from build123d import *

# Parameters (mm, degrees)
PAD_DEPTH            = 6.5
POCKET_DEPTH         = 6
SKETCH002_R          = 13.5
POCKET001_DEPTH      = 1
SKETCH003_W          = 5.45
SKETCH003_H          = 6.5
PAD001_DEPTH         = 3.5
POCKET002_DEPTH      = 10
SKETCH010_W          = 4
SKETCH010_H          = 6.5
PAD002_DEPTH         = 3.5
POCKET005_DEPTH      = 10
SKETCH015_R          = 2.2
SKETCH015_R_2        = 1.025
PAD003_DEPTH         = 2
POCKET009_DEPTH      = 4
POCKET010_DEPTH      = 4
PAD004_DEPTH         = 4
POCKET013_DEPTH      = 12.201
POCKET013_DEPTH_BACK = 36.201
SKETCH022_R          = 0.6
POCKET014_DEPTH      = 2
SKETCH023_R          = 0.6
POCKET015_DEPTH      = 2
SKETCH024_R          = 13.5
PAD005_DEPTH         = 1
SKETCH025_R          = 20.45
SKETCH025_R_2        = 19.85
POCKET016_DEPTH      = 0.3
SKETCH026_R          = 1
POCKET017_DEPTH      = 5


with BuildPart() as part:
    # Sketch → Pad (new body)
    with BuildSketch(Plane.XY):
        with BuildLine():
            Line((-22.5019915649, 16), (-22.5019915649, -16))
            Line((-22.5019915649, -16), (-16.2858834578, -17.9))
            ThreePointArc((-16.2858834578, -17.9), (-0.4552796053, -24.1957169863), (15.6009615088, -18.5))
            Line((15.6009615088, -18.5), (24.5395016581, -17.45))
            Line((24.5395016581, 17.45), (24.5395016581, -17.45))
            Line((15.6009615088, 18.5), (24.5395016581, 17.45))
            ThreePointArc((15.6009615088, 18.5), (-0.4552796053, 24.1957169863), (-16.2858834578, 17.9))
            Line((-22.5019915649, 16), (-16.2858834578, 17.9))
        make_face()
    extrude(amount=PAD_DEPTH)

    # Sketch001 → Pocket (cut)
    with BuildSketch(Plane.XY):
        with BuildLine():
            Line((-14.8539557021, 16.9), (-21.2122180433, 15.55))
            Line((-21.2122180433, 15.55), (-21.2122180433, -15.55))
            Line((-21.2122180433, -15.55), (-14.8539557021, -16.9))
            ThreePointArc((-14.8539557021, -16.9), (-0.0760301383, -22.4998715423), (14.739402973, -17))
            Line((14.739402973, -17), (23.6191552218, -16.4))
            Line((23.6191552218, 16.4), (23.6191552218, -16.4))
            Line((14.739402973, 17), (23.6191552218, 16.4))
            ThreePointArc((14.739402973, 17), (-0.0760301383, 22.4998715423), (-14.8539557021, 16.9))
        make_face()
    extrude(amount=POCKET_DEPTH, mode=Mode.SUBTRACT)

    # Sketch002 (on Face19 of Pocket) → Pocket001 (cut)
    with BuildSketch(Plane(origin=(0, 0, 6), x_dir=(1, 0, 0), z_dir=(0, 0, -1))):
        Circle(SKETCH002_R)
    extrude(amount=-POCKET001_DEPTH, mode=Mode.SUBTRACT)

    # Sketch003 (on Face7 of Pad) → Pad001 (join)
    with BuildSketch(Plane.YZ.offset(24.5395016581)):
        with Locations((-14.725, 3.25)):
            Rectangle(SKETCH003_W, SKETCH003_H)
        with Locations((14.725, 3.25)):
            Rectangle(SKETCH003_W, SKETCH003_H)
    extrude(amount=PAD001_DEPTH)

    # Sketch006 (on Face22 of Pad001) → Pocket002 (cut)
    with BuildSketch(Plane.XY.offset(6.5)):
        with BuildLine():
            ThreePointArc((24.5395016581, 17.45), (26.1592830786, 16.2095505764), (28.0395016581, 15.4176006311))
            Line((28.0395016581, 17.45), (28.0395016581, 15.4176006311))
            Line((28.0395016581, 17.45), (24.5395016581, 17.45))
        make_face()
        with BuildLine():
            ThreePointArc((28.0395016581, -15.4176006311), (26.1592830786, -16.2095505765), (24.5395016581, -17.4500000001))
            Line((28.0395016581, -17.45), (24.5395016581, -17.4500000001))
            Line((28.0395016581, -15.4176006311), (28.0395016581, -17.45))
        make_face()
    extrude(amount=-POCKET002_DEPTH, mode=Mode.SUBTRACT)

    # Sketch010 (on Face3 of Pad) → Pad002 (join)
    with BuildSketch(Plane(origin=(-22.5019915649, 0, 0), x_dir=(0, -1, 0), z_dir=(-1, 0, 0))):
        with Locations((-14, 3.25)):
            Rectangle(SKETCH010_W, SKETCH010_H)
        with Locations((14, 3.25)):
            Rectangle(SKETCH010_W, SKETCH010_H)
    extrude(amount=PAD002_DEPTH)

    # Sketch011 (on Face28 of Pad002) → Pocket005 (cut)
    with BuildSketch(Plane.XY.offset(6.5)):
        Polygon((-26.0019915649, 16), (-22.5019915649, 16), (-26.0019915649, 14.5), align=None)
        Polygon((-22.5019915649, -16), (-26.0019915649, -14.5), (-26.0019915649, -16), align=None)
    extrude(amount=-POCKET005_DEPTH, mode=Mode.SUBTRACT)

    # Sketch015 (on Face19 of Pocket) → Pad003 (join)
    with BuildSketch(Plane(origin=(0, 0, 6), x_dir=(1, 0, 0), z_dir=(0, 0, -1))):
        with Locations((-18.42, 13.32)):
            Circle(SKETCH015_R)
        with Locations((-18.42, 13.32)):
            Circle(SKETCH015_R_2, mode=Mode.SUBTRACT)
        with Locations((7.27, 18.56)):
            Circle(SKETCH015_R)
        with Locations((7.27, 18.56)):
            Circle(SKETCH015_R_2, mode=Mode.SUBTRACT)
        with Locations((5.37, -19.79)):
            Circle(SKETCH015_R)
        with Locations((5.37, -19.79)):
            Circle(SKETCH015_R_2, mode=Mode.SUBTRACT)
        with Locations((-18.42, -13.32)):
            Circle(SKETCH015_R)
        with Locations((-18.42, -13.32)):
            Circle(SKETCH015_R_2, mode=Mode.SUBTRACT)
    extrude(amount=PAD003_DEPTH)

    # Sketch016 (on Face4 of Pocket) → Pocket009 (cut)
    with BuildSketch(Plane(origin=(0, 0, 0), x_dir=(1, 0, 0), z_dir=(0, 0, -1))):
        with BuildLine():
            Line((-4.9992330338, 23.6779996848), (-5.0007669662, 21.9372361465))
            ThreePointArc((5.0007669662, 21.9372361465), (0, 22.5), (-5.0007669662, 21.9372361465))
            Line((5.0007669662, 23.6776757675), (5.0007669662, 21.9372361465))
            ThreePointArc((5.0007669662, 23.6776757675), (0.00078388, 24.1999999873), (-4.9992330338, 23.6779996848))
        make_face()
    extrude(amount=-POCKET009_DEPTH, mode=Mode.SUBTRACT)

    # Sketch017 (on Face4 of Pocket) → Pocket010 (cut)
    with BuildSketch(Plane(origin=(0, 0, 0), x_dir=(1, 0, 0), z_dir=(0, 0, -1))):
        with BuildLine():
            ThreePointArc((-3.2541322314, -22.2634369184), (0, -22.5), (3.2541322314, -22.2634369184))
            Line((3.2541322314, -22.2634369184), (3.5, -23.9455632634))
            ThreePointArc((-3.5, -23.9455632634), (0, -24.2), (3.5, -23.9455632634))
            Line((-3.2541322314, -22.2634369184), (-3.5, -23.9455632634))
        make_face()
        with BuildLine():
            ThreePointArc((-13.9498796389, -17.6536358312), (-11.25, -19.4855715851), (-8.3135572795, -20.9077680626))
            Line((-8.3135572795, -20.9077680626), (-8.9416927184, -22.487466094))
            ThreePointArc((-15.0038705449, -18.987466094), (-12.1, -20.9578147716), (-8.9416927184, -22.487466094))
            Line((-13.9498796389, -17.6536358312), (-15.0038705449, -18.987466094))
        make_face()
        with BuildLine():
            ThreePointArc((8.3135572795, -20.9077680626), (11.25, -19.4855715851), (13.9498796389, -17.6536358312))
            Line((13.9498796389, -17.6536358312), (15.0038705449, -18.987466094))
            ThreePointArc((8.9416927184, -22.487466094), (12.1, -20.9578147716), (15.0038705449, -18.987466094))
            Line((8.3135572795, -20.9077680626), (8.9416927184, -22.487466094))
        make_face()
    extrude(amount=-POCKET010_DEPTH, mode=Mode.SUBTRACT)

    # Sketch018 (on Face8 of Pocket005) → Pad004 (join)
    with BuildSketch(Plane(origin=(0, 0, 0), x_dir=(1, 0, 0), z_dir=(0, 0, -1))):
        Polygon((-26.0019915649, 14.5), (-26.0019915649, 12), (-22.5019915649, 12), (-22.5019915649, 16), align=None)
        Polygon((-26.0019915649, -12), (-22.5019915649, -12), (-22.5019915649, -16), (-26.0019915649, -14.5), align=None)
        with BuildLine():
            Line((24.5395016581, 17.4500000001), (24.5395016581, 12))
            Line((28.0395016581, 12), (24.5395016581, 12))
            Line((28.0395016581, 15.4176006311), (28.0395016581, 12))
            ThreePointArc((24.5395016581, 17.4500000001), (26.1592830786, 16.2095505765), (28.0395016581, 15.4176006311))
        make_face()
        with BuildLine():
            Line((24.5395016581, -12), (24.5395016581, -17.45))
            ThreePointArc((28.0395016581, -15.4176006311), (26.1592830786, -16.2095505764), (24.5395016581, -17.45))
            Line((28.0395016581, -12), (28.0395016581, -15.4176006311))
            Line((24.5395016581, -12), (28.0395016581, -12))
        make_face()
    extrude(amount=PAD004_DEPTH)

    # Sketch021 (on Face50 of Pad004) → Pocket013 (cut, two sides)
    with BuildSketch(Plane(origin=(0, -12, 0), x_dir=(-1, 0, 0), z_dir=(0, 1, 0))) as pocket013_sk:
        with BuildLine():
            Line((-24.5395016581, -4), (-24.5395016581, -2))
            ThreePointArc((-26.5395016581, -4), (-25.1252880957, -3.4142135624), (-24.5395016581, -2))
            Line((-24.5395016581, -4), (-26.5395016581, -4))
        make_face()
        with BuildLine():
            Line((22.5019915649, -4), (22.5019915649, -2))
            ThreePointArc((22.5019915649, -2), (23.0877780026, -3.4142135624), (24.5019915649, -4))
            Line((22.5019915649, -4), (24.5019915649, -4))
        make_face()
        with BuildLine():
            Line((-28.0395016581, 0), (-28.0395016581, 6.5))
            Line((-28.0395016581, 6.5), (-24.5395016581, 6.5))
            ThreePointArc((-24.5395016581, 6.5), (-27.1088837932, 3.6912057651), (-28.0395016581, 0))
        make_face()
        with BuildLine():
            Line((26.0019915649, 6.5), (26.0019915649, 0))
            ThreePointArc((26.0019915649, 0), (25.0713737, 3.6912057651), (22.5019915649, 6.5))
            Line((26.0019915649, 6.5), (22.5019915649, 6.5))
        make_face()
    extrude(amount=-POCKET013_DEPTH, mode=Mode.SUBTRACT)
    extrude(pocket013_sk.sketch, amount=POCKET013_DEPTH_BACK, mode=Mode.SUBTRACT)

    # Sketch022 (on Face66 of Pocket013) → Pocket014 (cut)
    with BuildSketch(Plane.XZ.offset(-12)):
        with Locations((-24.7019915649, -2.7)):
            Circle(SKETCH022_R)
        with Locations((26.7395016581, -2.7)):
            Circle(SKETCH022_R)
    extrude(amount=-POCKET014_DEPTH, mode=Mode.SUBTRACT)

    # Sketch023 (on Face49 of Pocket014) → Pocket015 (cut)
    with BuildSketch(Plane(origin=(0, -12, 0), x_dir=(-1, 0, 0), z_dir=(0, 1, 0))):
        with Locations((-26.7395016581, -2.7)):
            Circle(SKETCH023_R)
        with Locations((24.7019915649, -2.7)):
            Circle(SKETCH023_R)
    extrude(amount=-POCKET015_DEPTH, mode=Mode.SUBTRACT)

    # Sketch024 (on Face16 of Pocket015) → Pad005 (join)
    with BuildSketch(Plane.XY.offset(6.5)):
        with BuildLine():
            ThreePointArc((-22.5019915649, -8.9050758341), (24.2, 0), (-22.5019915649, 8.9050758341))
            Line((-22.5019915649, 8.9050758341), (-22.5019915649, -8.9050758341))
        make_face()
        Circle(SKETCH024_R, mode=Mode.SUBTRACT)
    extrude(amount=PAD005_DEPTH)

    # Sketch025 (on Face42 of Pad005) → Pocket016 (cut)
    with BuildSketch(Plane.XY.offset(7.5)):
        Circle(SKETCH025_R)
        Circle(SKETCH025_R_2, mode=Mode.SUBTRACT)
    extrude(amount=-POCKET016_DEPTH, mode=Mode.SUBTRACT)

    # Sketch026 (on DatumPlane) → Pocket017 (cut)
    with BuildSketch(Plane.XZ.offset(25)):
        with Locations((-6.5, 4.8)):
            Circle(SKETCH026_R)
    extrude(amount=-POCKET017_DEPTH, mode=Mode.SUBTRACT)


solid = part.part
Read the model definition and answer for the solid it produces. Units are mm, in the model's axes. A direction names the side the tool comes from. Coordinates: 2 decimals unless noted, no trailing zeros. Loops run counter-clockwise (first coordinate to the right, second up) from the corner with the lowest first, then second, coordinate; pieces in that order, holes last. Notation, with made-up numbers: (65.25, 81) -> (120.25, 81) arc R17 ccw to (120.25, 99) -> close; hole circle Ø6 at (6, -9). An arc over 180 degrees is marked (long way). Answer in a Markdown table with one row per item.
Item 1: A cutting plane is placed at D-D on x = -6.5. Determine the outline of the cut face in (y, z).
Returned:
| item | result |
|---|---|
| outline | (-23.31, 0) -> (-21.54, 0) -> (-21.54, 3.8) -> (-23.31, 3.8) -> close; (-23.31, 5.8) -> (-21.54, 5.8) -> (-21.54, 6) -> (-11.83, 6) -> (-11.83, 7.5) -> (-18.76, 7.5) -> (-18.76, 7.2) -> (-19.39, 7.2) -> (-19.39, 7.5) -> (-23.31, 7.5) -> close; (11.83, 6) -> (21.54, 6) -> (21.54, 0) -> (23.31, 0) -> (23.31, 7.5) -> (19.39, 7.5) -> (19.39, 7.2) -> (18.76, 7.2) -> (18.76, 7.5) -> (11.83, 7.5) -> close |
Item 2: A cutting plane is placed at B-B on z = -0.75. Determine the outline of the cut face in (x, y), plus the area to 3 significant figures.
Returned:
| item | result |
|---|---|
| outline | (-26, -14.5) -> (-22.5, -16) -> (-22.5, -12) -> (-26, -12) -> close; (-26, 12) -> (-22.5, 12) -> (-22.5, 16) -> (-26, 14.5) -> close; (24.54, -17.45) arc R8.03 cw to (28.04, -15.42) -> (28.04, -12) -> (24.54, -12) -> close; (24.54, 12) -> (28.04, 12) -> (28.04, 15.42) arc R8.03 cw to (24.54, 17.45) -> close |
| area | 52.4 mm^2 |
Item 3: For a pull along Y with two mould halves and no side action, classify faces 1 (the flat face through (-24.23, -15.26, 0.16)), 2 (the flat face through (19.117, -16.704, 2.958)), 3 (the flat face through (28.04, 14, -2)) as released by +Y, released by -Y, zero draft, split by the parting line, or undercut.
Returned:
| item | result |
|---|---|
| face 1 | released by -Y |
| face 2 | undercut |
| face 3 | zero draft |
Item 4: A cutting plane is placed at A-A on x = 0. Determine the outline of the cut face in (y, z).
Returned:
| item | result |
|---|---|
| outline | (-24.2, 4) -> (-22.5, 4) -> (-22.5, 6) -> (-13.5, 6) -> (-13.5, 7.5) -> (-19.85, 7.5) -> (-19.85, 7.2) -> (-20.45, 7.2) -> (-20.45, 7.5) -> (-24.2, 7.5) -> close; (13.5, 6) -> (22.5, 6) -> (22.5, 4) -> (24.2, 4) -> (24.2, 7.5) -> (20.45, 7.5) -> (20.45, 7.2) -> (19.85, 7.2) -> (19.85, 7.5) -> (13.5, 7.5) -> close |
Item 5: For faces 4 (the flat face through (-24, -12, 0)), 5 (the flat face through (-18.078, -16.216, 2.958)), 6 (the flat face through (-25, 14, -3)), 7 (the flat face through (26, 12, 1)), determine the directions among +Z, -Z, +X, -X, +Y, -Y from which every point of the face is accessible in a straight line to the end or side of a thin tool.
Returned:
| item | result |
|---|---|
| face 4 | +Z, -Z, -X |
| face 5 | -Z |
| face 6 | none |
| face 7 | +Z, -Z, +X |
Item 6: Straight lines are drawn through the part: line 1 along X through (y, z) = (-13.32, 5.1) (3 decimals); line 2 along Z through (x, y) = (-6.5, -22.5); line 3 along X through (y, z) = (-0.5, 7). For each, find the intervals that lie inside material, in ascending order. Write a range as [from, to].
Returned:
| item | result |
|---|---|
| line 1 | x = [-24.099, -21.212], [-20.62, -19.445], [-17.395, -16.22], [23.619, 26.137] |
| line 2 | z = [0, 3.8], [5.8, 7.5] |
| line 3 | x = [-22.5, -13.49], [13.49, 24.19] |
Item 7: Each of these flat-tipped pins is pushed along its axis until it touches: P1, Ø1, axis at x = 26.74, z = -2.7, coming from the +Y side; P2, Ø6, axis at x = 18.5, y = -17.5, coming from the -Z side; P3, Ø1, axis at x = 21.5, z = 0.5, coming from the +Y side; P4, Ø4, axis at x = 5.5, z = -2.5, coming from the +Y side. Where does it stop, or does it pass through?
Returned:
| item | result |
|---|---|
| P1 | stops at y = 16.16 |
| P2 | stops at z = 0 |
| P3 | stops at y = 17.87 |
| P4 | passes through |
Item 8: A cutting plane is placed at C-C on y = 0. Determine the outline of the cut face in (x, z).
Returned:
| item | result |
|---|---|
| outline | (-22.5, 0) -> (-21.21, 0) -> (-21.21, 6) -> (-13.5, 6) -> (-13.5, 7.5) -> (-19.85, 7.5) -> (-19.85, 7.2) -> (-20.45, 7.2) -> (-20.45, 7.5) -> (-22.5, 7.5) -> close; (13.5, 6) -> (23.62, 6) -> (23.62, 0) -> (24.54, 0) -> (24.54, 6.5) -> (24.2, 6.5) -> (24.2, 7.5) -> (20.45, 7.5) -> (20.45, 7.2) -> (19.85, 7.2) -> (19.85, 7.5) -> (13.5, 7.5) -> close |
